Autodesk Inventor part; units mm, degrees
ref_plane "YZ Plane" through (0, 0, 0) normal (1, 0, 0) x (0, 1, 0)
ref_plane "XZ Plane" through (0, 0, 0) normal (0, 1, 0) x (-1, 0, 0)
ref_plane "XY Plane" through (0, 0, 0) normal (0, 0, 1) x (1, 0, 0)
sketch "Skizze1" plane through (0, 0, 0) normal (0, 0, 1) x (1, 0, 0)
  line L0 (-2.5, 1.4434) -> (0, 2.8868)
  line L1 (0, 2.8868) -> (2.5, 1.4434)
  line L2 (2.5, 1.4434) -> (2.5, -1.4434)
  line L3 (2.5, -1.4434) -> (0, -2.8868)
  line L4 (0, -2.8868) -> (-2.5, -1.4434)
  line L5 (-2.5, -1.4434) -> (-2.5, 1.4434)
  point P0 (0, 0)
  point P1 (0, 0)
  point P2 (0, 0)
  dimension "d2" = 5
extrude "Extrusion1" add sketch "Skizze1" along normal mid plane 4.5
sketch "Skizze3" plane through (0, 0, 2.25) normal (0, 0, 1) x (1, 0, 0)
  point P0 (0, 0)
  point P1 (0, 0)
hole "Bohrung1" at (0, 0, 2.25) direction (0, 0, -1) diameter 2.459 depth 8.8 tip angle 118
sketch "Skizze4" plane through (0, 0, -2.25) normal (0, 0, -1) x (-1, 0, 0)
  circle A0 centre (0, 0) radius 1.5
  dimension "d17" = 3
extrude "Extrusion3" add sketch "Skizze4" along normal blind 6
thread "Gewinde2"
chamfer "Fase1" distance 0.25 angle 45 1 edges at (1.5, 0, -8.25)
properties part number "standoff (1466814)"
Source: CAD feature listing. Evaluate the final solid. Frame: model axes, mm. A direction names the side the tool comes from. Round coordinates to 2 decimals unless told otherwise and drop trailing zeros. Loops run counter-clockwise (first coordinate to the right, second up) from the corner with the lowest first, then second, coordinate; pieces in that order, holes last.
Q1. Access query for faces 4 (the face through (1.5, -0.07, -5.08)), 5 (the face through (-1.267, 2.155, -0.031)), 6 (the face through (0, 0, -2.25)). Directions: +Z, -Z, +X, -X, +Y, -Y. A direction counts if a zero-diameter tool reaches every point of the face in a straight line with its end or side. Return the directions, or none.
Q2. Section C-C, the plane z = -3.25. Return loops of the section in (x, y).
Q3. Section B-B, the plane y = 0. Return loops of the section in (x, z), plus the area to 3 significant figures.
Q4. Ray query, line 1 (X direction, y = 0, z = 0.9); line 2 (Z direction, x = -0.95, y = 1.55); line 3 (Z direction, x = -0.85, y = 0.85). Return the intervals inside material, ascending.
Q5. Section D-D, the plane x = -1.85. Return loops of the section in (y, z), plus the area to 3 significant figures.
Q6. First-contact query: P1, Ø1, axis at x = -2, z = 0.5, coming from the +Y side; P2, Ø1.5, axis at y = 0.5, z = -7, coming from the +X side; P3, Ø1, axis at x = -1.5, z = -6.5, coming from the +Y side. Flat tips, straight axial feed; report the tip coordinate or a pass-through.
Q7. Mould query, pull axis X, two halves, no side actions, for faces 1 (the face through (0.748, 0.976, -0.031)), 2 (the face through (-1.15, -1.24, -2.25)), 3 (the face through (1.267, -2.155, -0.031)). Classes: pulls with the +X half, pulls with the -X half, needs draft (parallel to the pull), parting line crosses it, or undercut.
Q8. Section A-A, the plane z = -1.5. Return loops of the section in (x, y), plus the area to 3 significant figures.
Solutions:
1. face 4: -Z
1. face 5: +Z, -Z, -X, +Y
1. face 6: +Z
2. outline: circle Ø3 at (0, 0)
3. outline: (-2.5, -2.25) - (-1.5, -2.25) - (-1.5, -8) - (-1.25, -8.25) - (1.25, -8.25) - (1.5, -8) - (1.5, -2.25) - (2.5, -2.25) - (2.5, 2.25) - (1.23, 2.25) - (1.23, -2.25) - (-1.23, -2.25) - (-1.23, 2.25) - (-2.5, 2.25) - close
3. area: 29.4 mm2
4. line 1: x = -2.5 to -1.23, 1.23 to 2.5
4. line 2: z = -2.25 to 2.25
4. line 3: z = -8.25 to -2.25
5. outline: (-1.82, -2.25) - (1.82, -2.25) - (1.82, 2.25) - (-1.82, 2.25) - close
5. area: 16.4 mm2
6. P1: stops at y = 2.02
6. P2: stops at x = 1.5
6. P3: stops at y = 1.12
7. face 1: undercut
7. face 2: needs draft
7. face 3: pulls with the +X half
8. outline: (-2.5, -1.44) - (0, -2.89) - (2.5, -1.44) - (2.5, 1.44) - (0, 2.89) - (-2.5, 1.44) - close; hole circle Ø2.46 at (0, 0)
8. area: 16.9 mm2
